Solid Edge part; units mm, degrees
sketch "Sketch1" plane through (0, 0, 0) normal (1, 0, 0) x (0, 1, 0)
  line L0 (-22.0921, 14.4671) -> (-22.0921, -5.3577)
  arc A0 (-22.0921, -5.3577) -> (-20.7015, -6.7483) centre (-20.7015, -5.3577) ccw
  line L1 (-20.7015, -6.7483) -> (-3.1627, -6.7483)
  arc A1 (-1.7721, -5.3577) -> (-3.1627, -6.7483) centre (-3.1627, -5.3577) cw
  line L2 (-1.7721, -5.3577) -> (-1.7721, 14.4671)
  arc A2 (-3.2811, 15.8527) -> (-1.7721, 14.4671) centre (-3.1627, 14.4671) cw
  arc A3 (-20.5831, 15.8527) -> (-22.0921, 14.4671) centre (-20.7015, 14.4671) ccw
  arc A4 (-3.2811, 15.8527) -> (-20.5831, 15.8527) centre (-11.9321, 117.0837) cw
extrude "Protrusion1" add sketch "Sketch1" along normal mid plane 8.636
fillet "Round_1" radius 1.27 4 edges at (4.318, -22.0921, 4.5547) (-4.318, -22.0921, 4.5547) (4.318, -1.7721, 4.5547) (-4.318, -1.7721, 4.5547)
sketch "Sketch2" plane through (0, -11.6781, -6.7483) normal (0, 0, -1) x (-1, 0, 0)
  circle A0 centre (0, 5.3086) radius 0.5
  circle A1 centre (0, -5.8166) radius 0.5
extrude "ExtrudedProtrusion_2" add sketch "Sketch2" along normal blind 2.54
For this review, take the finished solid that the model builds, in its own axes (mm). A direction names the side the tool comes from. Give positions to 0.01 mm unless a question says otherwise; leave off trailing zeros. Write each loop counter-clockwise with the first axis right and the second up, starting at its lowest first coordinate (ties: lowest second). Pieces come first, ordered by that corner, then holes.
Item 1: Take a section at C-C (x = -2.25). Give the boundary of the cut face in (y, z).
Item 2: Insertion check: P1, Ø2.5, axis at x = 0.5, y = -13.5, coming from the -Z side. The pin has a flat end and moves straight along its axis. Give the tip position at first contact, or say it passes through.
Item 3: Take a section at B-B (y = -15). Give the boundary of the cut face in (x, z), and give its area (3 significant figures).
Item 4: Take a section at A-A (x = 0). Give the boundary of the cut face in (y, z), and give its area (3 significant figures).
Item 5: The part is to be moulded in two halves that separate along Y. For faces 3 (the face through (0, -17.5, -9.288)), 4 (the face through (-0.06, -11.811, 15.484)), 5 (the face through (3.936, -21.73, 4.713)), say which applies: +Y half, -Y half, draft (parallel to the pull), parting line (faces both ways), or undercut.
Item 6: Wall thickness on probe 1 along Z at (x, y) = (0.75, -12.5); probe 2 along Z at (x, y) = (3, -3); probe 3 along Y at (x, z) = (3.5, -5.25): over which ranges is each line inside the solid? List them lowest first.
Item 7: Take a section at D-D (y = -9.25). Give the boundary of the cut face in (x, z).
Item 8: Machinability: for faces 1 (the face through (-4.318, -12, 4)), 2 (the face through (0.065, -6.865, -8.001)), which of the approach directions +Z, -Z, +X, -X, +Y, -Y give a long, thin tool a straight path to every point of the face, cutting with its end or side? Answer none if there is none.
Established:
1. outline: (-22.09, -5.36) arc R1.39 ccw to (-20.7, -6.75) - (-3.16, -6.75) arc R1.39 ccw to (-1.77, -5.36) - (-1.77, 14.47) arc R1.39 ccw to (-3.28, 15.85) arc R101.6 cw to (-20.58, 15.85) arc R1.39 ccw to (-22.09, 14.47) - close
2. P1: stops at z = -6.75
3. outline: (-4.32, -6.75) - (4.32, -6.75) - (4.32, 15.53) - (-4.32, 15.53) - close
3. area: 192 mm2
4. outline: (-22.09, -5.36) arc R1.39 ccw to (-20.7, -6.75) - (-17.99, -6.75) - (-17.99, -9.29) - (-16.99, -9.29) - (-16.99, -6.75) - (-6.87, -6.75) - (-6.87, -9.29) - (-5.87, -9.29) - (-5.87, -6.75) - (-3.16, -6.75) arc R1.39 ccw to (-1.77, -5.36) - (-1.77, 14.47) arc R1.39 ccw to (-3.28, 15.85) arc R101.6 cw to (-20.58, 15.85) arc R1.39 ccw to (-22.09, 14.47) - close
4. area: 458 mm2
5. face 3: draft
5. face 4: undercut
5. face 5: -Y half
6. probe 1: z = -6.75 to 15.49
6. probe 2: z = -6.74 to 15.85
6. probe 3: y = -22.01 to -1.86
7. outline: (-4.32, -6.75) - (4.32, -6.75) - (4.32, 15.52) - (-4.32, 15.52) - close
8. face 1: +Z, -Z, -X, +Y, -Y
8. face 2: -Z
